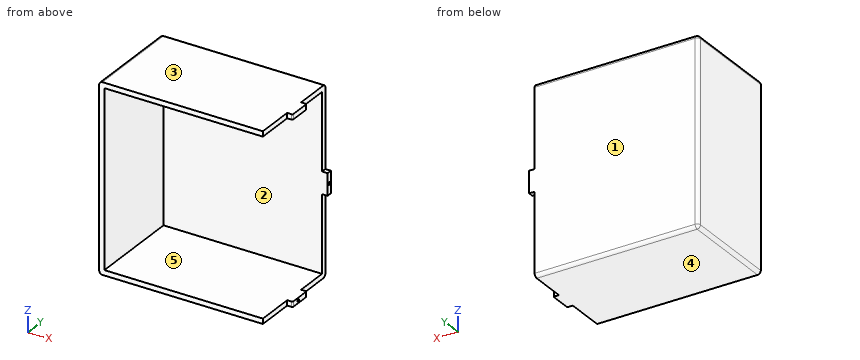
Autodesk Inventor part; units mm, degrees
ref_plane "YZ Plane" through (0, 0, 0) normal (1, 0, 0) x (0, 1, 0)
ref_plane "XZ Plane" through (0, 0, 0) normal (0, 1, 0) x (-1, 0, 0)
ref_plane "XY Plane" through (0, 0, 0) normal (0, 0, 1) x (1, 0, 0)
sketch "Sketch1" plane through (0, 0, 0) normal (0, 1, 0) x (-1, 0, 0)
  line L0 (0, 0) -> (-150, 0)
  line L1 (0, -170) -> (0, 0)
  line L2 (0, -170) -> (-150, -170)
  line L3 (-150, -170) -> (-150, -95)
  line L4 (-150, -95) -> (-155, -95)
  line L5 (-155, -95) -> (-155, -75)
  line L6 (-155, -75) -> (-150, -75)
  line L7 (-150, -75) -> (-150, 0)
  dimension "d28" = 150
  dimension "d29" = 170
  dimension "d30" = 5
  dimension "d31" = 5
  dimension "d32" = 75
  dimension "d33" = 75
  dimension "d34" = 20
  dimension "d35" = 150
extrude "Extrusion1" add sketch "Sketch1" along normal blind 4.7625
sketch "Sketch2" plane through (0, 0, 0) normal (0, -1, 0) x (1, 0, 0)
  line L0 (0, 0) -> (150, 0)
  line L1 (0, 0) -> (4.7625, 0)
  line L2 (150, -170) -> (0, -170)
  line L3 (0, 0) -> (0, -170)
  line L4 (0, -170) -> (4.7625, -170)
  line L5 (4.7625, -170) -> (4.7625, 0)
  point P0 (0, -90)
  point P1 (4.7625, -90)
  dimension "d10" = 90
  dimension "d11" = 4.7625
extrude "Extrusion2" add sketch "Sketch2" along normal blind 85.2375
sketch "Sketch3" plane through (0, 0, 0) normal (0, -1, 0) x (1, 0, 0)
  line L0 (150, -95) -> (150, -170)
  line L1 (150, -170) -> (150, -165.2375)
  line L2 (150, -165.2375) -> (4.7625, -165.2375)
  line L3 (4.7625, 0) -> (4.7625, -170)
  line L4 (150, -170) -> (4.7625, -170)
  line L5 (4.7625, -170) -> (4.7625, -165.2375)
  line L6 (150, -170) -> (4.7625, -170)
  line L7 (150, -170) -> (150, -165.2375)
  point P0 (0, 0)
  dimension "d36" = 4.7625
sketch "Sketch4" plane through (0, 0, 0) normal (0, -1, 0) x (1, 0, 0)
  line L0 (150, 0) -> (150, -35)
  line L1 (150, 0) -> (150, -4.7625)
  line L2 (150, -4.7625) -> (4.7625, -4.7625)
  line L3 (4.7625, -85.2375) -> (4.7625, 0)
  line L4 (4.7625, 0) -> (150, 0)
  line L5 (4.7625, 0) -> (150, 0)
  line L6 (4.7625, -4.7625) -> (4.7625, 0)
  point P0 (0, 0)
  dimension "d17" = 4.7625
extrude "Extrusion4" add sketch "Sketch4" along normal blind 85.2375
sketch "Sketch6" plane through (0, 4.7625, 0) normal (0, 0, 1) x (1, 0, 0)
  line L0 (150, -4.7625) -> (150, -90)
  line L1 (150, -4.7625) -> (150, -90)
  line L2 (150, -90) -> (0, -90)
  line L3 (0, 0) -> (150, 0)
  line L4 (150, -55) -> (155, -55)
  line L5 (155, -55) -> (155, -35)
  line L6 (155, -35) -> (150, -35)
  line L7 (150, -35) -> (150, -55)
  point P0 (0, -4.7625)
  point P1 (150, -31.3995)
  dimension "d90" = 20
  dimension "d91" = 5
  dimension "d92" = 35
  dimension "d93" = 35
extrude "Extrusion6" add sketch "Sketch6" against normal blind 4.7625
extrude "Extrusion7" add sketch "Sketch3" along normal blind 85.2375
sketch "Sketch7" plane through (150, 4.7625, -170) normal (0, 0, -1) x (-1, 0, 0)
  line L0 (0, -4.7625) -> (0, -90)
  line L1 (0, -55) -> (-5, -55)
  line L2 (-5, -55) -> (-5, -35)
  line L3 (-5, -35) -> (0, -35)
  line L4 (0, -35) -> (0, -55)
  line L5 (150, -90) -> (0, -90)
  line L6 (0, 0) -> (150, 0)
  point P0 (150, -4.7625)
  point P1 (-5, -31.3995)
  dimension "d74" = 20
  dimension "d75" = 5
  dimension "d76" = 35
  dimension "d77" = 35
extrude "Extrusion8" add sketch "Sketch7" against normal blind 4.7625
fillet "Fillet3" radius 3 1 edges at (0, 4.7625, -85)
fillet "Fillet4" radius 3 6 edges at (0.8787, 3.8838, -170) (0, -41.7375, -170) (76.5, 4.7625, -170) (0.8787, 3.8838, 0) (0, -41.7375, 0) (76.5, 4.7625, 0)
hole "Hole3" at (155, 2.4466, -85.2501) direction (-1, 0, 0) diameter 2.5 depth 5 tip angle 118
hole "Hole4" at (155, -42.3344, -167.7364) direction (-1, 0, 0) diameter 2.5 depth 5 tip angle 118
fillet "Fillet5" radius 1 2 edges at (155, -50.2375, -167.6188) (155, -30.2375, -167.6188)
fillet "Fillet6" radius 1 2 edges at (155, -50.2375, -2.3813) (155, -30.2375, -2.3813)
properties part number "OpticalDeviceObjectPart"
Model file for the job. Use its own axes, mm. Face numbers are marked on the shaded views. A direction names the side the tool comes from. Round coordinates to 2 decimals unless told otherwise and drop trailing zeros. Order: outer loops, then holes, each group sorted by start corner. A loop starts at its lowest first (then second) coordinate and runs counter-clockwise, first axis right, second up. Notation, with made-up numbers: (50.5, 74) -> (87.5, 74) arc R23 ccw to (87.5, 83) -> close; hole circle Ø5 at (55.5, 72.25). An arc over 180 degrees is marked (long way). Use one line per item in the form item = value.
Item 1: Cut at C-C, the plane z = -89.5. Write the cut outline in (x, y).
Returned:
outline = (0, -85.24) -> (4.76, -85.24) -> (4.76, 0) -> (155, 0) -> (155, 4.76) -> (3, 4.76) arc R3 ccw to (0, 1.76) -> close
Item 2: Drill centre lines: line 1 (Z direction, x = 127, y = -19.5); line 2 (X direction, y = -44.5, z = -65). Where is each one in solid material? Low to high.
Returned:
line_1 = -170 to -165.24, -4.76 to 0
line_2 = 0 to 4.76
Item 3: Flat gauge pins, fed straight in: pin 1 Ø1.2 at (x, z) = (152, -3.5) entering from -Y; pin 2 Ø2 at (x, z) = (39, -137) entering from -Y; pin 3 Ø4 at (x, y) = (152.5, 3.5) entering from +Z. Where does each tip first touch, or does it go through?
Returned:
pin_1 = -50.24
pin_2 = 0
pin_3 = -75
Item 4: Cut at D-D, the plane z = -153.5. Write the cut outline in (x, y), and give its area (3 significant figures).
Returned:
outline = (0, -85.24) -> (4.76, -85.24) -> (4.76, 0) -> (150, 0) -> (150, 4.76) -> (3, 4.76) arc R3 ccw to (0, 1.76) -> close
area = 1,120 mm^2
Item 5: Pull direction Z, two halves, no side cores. Call the marked faces 1, 2 and 3: released by +Z, released by -Z, zero draft, split by the parting line, or undercut.
Returned:
face_1 = zero draft
face_2 = undercut
face_3 = released by +Z
Item 6: Cut at A-A, the plane x = 86. Write the cut outline in (y, z), and give its area (3 significant figures).
Returned:
outline = (-85.24, -170) -> (1.76, -170) arc R3 ccw to (4.76, -167) -> (4.76, -3) arc R3 ccw to (1.76, 0) -> (-85.24, 0) -> (-85.24, -4.76) -> (0, -4.76) -> (0, -165.24) -> (-85.24, -165.24) -> close
area = 1,620 mm^2
Item 7: Cut at B-B, the plane y = -59.5. Write the cut outline in (x, z), and give its area (3 significant figures).
Returned:
outline = (0, -167) arc R3 ccw to (3, -170) -> (150, -170) -> (150, -165.24) -> (4.76, -165.24) -> (4.76, -4.76) -> (150, -4.76) -> (150, 0) -> (3, 0) arc R3 ccw to (0, -3) -> close
area = 2,190 mm^2
Item 8: Tool access for the marked faces 4 and 5: list every direction of +Z, -Z, +X, -X, +Y, -Y with a clear straight run to the whole face (end or side of a thin tool).
Returned:
face_4 = -Z, +X, -X, +Y, -Y
face_5 = +X, -Y
